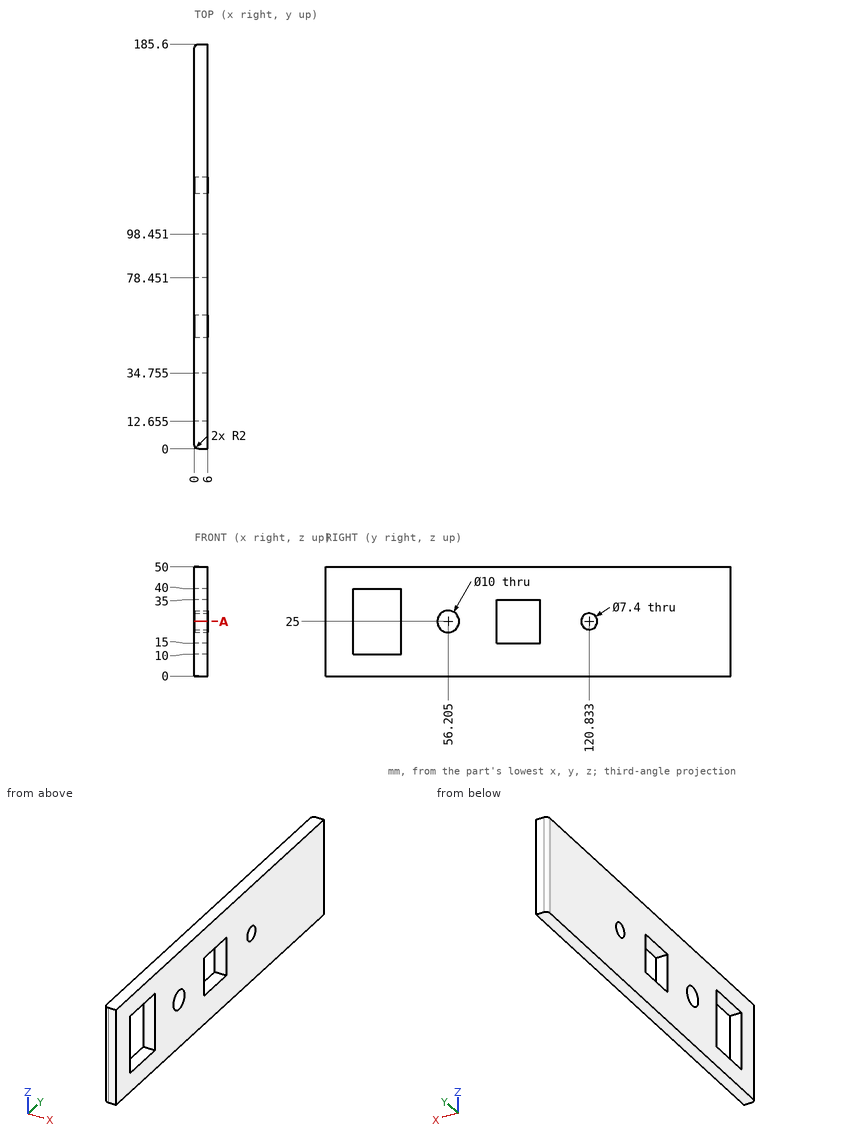
Design review of the part shown in the three views and the two pictorial views. Dimensions are in mm from the part's minimum x, y and z. Coordinates: 2 decimals unless noted, no trailing zeros. Order: outer loops, then holes, each group sorted by start corner. A loop starts at its lowest first (then second) coordinate and runs counter-clockwise, first axis right, second up.
1) Clearance check with a flat-ended pin moving along its axis: pin 1 (8 mm diameter, centred on y = 56.21, z = 25, fed in from -X). State where the tip first meets the part, or that it passes through.
2) Take a section at A-A, the plane z = 25. Give the boundary of the cut face in (x, y) (1 decimal).
3) Wall thickness on line 1 along Z through (x, y) = (5.75, 20.5); line 2 along Z through (x, y) = (1.65, 87); line 3 along Y through (x, z) = (1.8, 8): over which ranges is each line inside the solid? List them lowest first.
Returned:
1. pin 1: passes through
2. outline: (0, 2) arc R2 ccw to (2, 0) - (6, 0) - (6, 12.7) - (0, 12.7) - close; (0, 34.8) - (6, 34.8) - (6, 51.2) - (0, 51.2) - close; (0, 61.2) - (6, 61.2) - (6, 78.5) - (0, 78.5) - close; (0, 98.5) - (6, 98.5) - (6, 117.1) - (0, 117.1) - close; (0, 124.5) - (6, 124.5) - (6, 185.6) - (2, 185.6) arc R2 ccw to (0, 183.6) - close
3. line 1: z = 0 to 10, 40 to 50
3. line 2: z = 0 to 15, 35 to 50
3. line 3: y = 0.01 to 185.59
